Work out the finished part from the listing and answer in its coordinate system (mm). A direction names the side the tool comes from. Coordinates: 2 decimals unless noted, no trailing zeros. Order: outer loops, then holes, each group sorted by start corner. A loop starts at its lowest first (then second) coordinate and runs counter-clockwise, first axis right, second up. Notation, with made-up numbers: M 66,-19.5 L 98,-19.5 A17 cw 98,-0.5 Z; hole C 28,43 d7. An arc over 180 degrees is marked long. Use a Markdown table: item, result.
from build123d import *

# Parameters (mm, degrees)
SKETCH1_R           = 9.2
BOSS_EXTRUDE1_DEPTH = 65
CUT_EXTRUDE2_START  = -3
SKETCH2_R           = 9.2
SKETCH2_R_2         = 7.5
CUT_EXTRUDE2_DEPTH  = 3
CUT_EXTRUDE3_START  = -1.5
SKETCH3_R           = 9.2
SKETCH3_R_2         = 8.419577465
CUT_EXTRUDE3_DEPTH  = 1.5


with BuildPart() as part:
    # Sketch1 → Boss-Extrude1 (new body)
    with BuildSketch(Plane.XY):
        Circle(SKETCH1_R)
    extrude(amount=BOSS_EXTRUDE1_DEPTH)

    # Sketch2 → Cut-Extrude2 (cut)
    with BuildSketch(Plane.XY.offset(65).offset(CUT_EXTRUDE2_START)):
        Circle(SKETCH2_R)
        Circle(SKETCH2_R_2, mode=Mode.SUBTRACT)
    extrude(amount=CUT_EXTRUDE2_DEPTH, mode=Mode.SUBTRACT)

    # Sketch3 → Cut-Extrude3 (cut)
    with BuildSketch(Plane.XY.offset(58).offset(CUT_EXTRUDE3_START)):
        Circle(SKETCH3_R)
        Circle(SKETCH3_R_2, mode=Mode.SUBTRACT)
    extrude(amount=CUT_EXTRUDE3_DEPTH, mode=Mode.SUBTRACT)


solid = part.part
1. Flat-ended cylindrical pins translate along their axes: P1, Ø10, axis at x = -6, z = 54, coming from the -Y side; P2, Ø5, axis at y = -6.5, z = 45.5, coming from the +X side; P3, Ø8, axis at y = -6, z = 35.5, coming from the +X side. Find the tip coordinate at first contact, or state that the pin passes through.
Answers below:
| item | result |
|---|---|
| P1 | y = -9.15 |
| P2 | x = 8.28 |
| P3 | x = 8.98 |
2. For a pull along Z with two mould halves and no side action, classify faces 3 (the face through (0, 0, 0)), 4 (the face through (-7.3, -5.6, 60)), 5 (the face through (8.03, 2.53, 57.24)) as +Z half, -Z half, draft (parallel to the pull), parting line (faces both ways), or undercut.
Answers below:
| item | result |
|---|---|
| face 3 | -Z half |
| face 4 | draft |
| face 5 | undercut |
3. Find the intervals of material crossed by probe 1 along Z at (x, y) = (-7.5, -5); probe 2 along X at (y, z) = (-0.5, 9.5); probe 3 along X at (y, z) = (-7.5, 3.5), in increasing order.
Answers below:
| item | result |
|---|---|
| probe 1 | 0 to 56.5, 58 to 62 |
| probe 2 | -9.19 to 9.19 |
| probe 3 | -5.33 to 5.33 |
4. Section B-B on x = -1.5 is taken. Determine the outline of the cut face in (y, z), then the cut area to 3 significant figures.
Answers below:
| item | result |
|---|---|
| outline | M -9.08,0 L 9.08,0 L 9.08,56.5 L 8.28,56.5 L 8.28,58 L 9.08,58 L 9.08,62 L 7.35,62 L 7.35,65 L -7.35,65 L -7.35,62 L -9.08,62 L -9.08,58 L -8.28,58 L -8.28,56.5 L -9.08,56.5 Z |
| area | 1,170 mm² |
5. Section C-C on z = 53 is taken. Determine the outline of the cut face in (x, y).
Answers below:
| item | result |
|---|---|
| outline | C 0,0 d18.4 |
6. For faces 1 (the face through (0, 0, 65)), 2 (the face through (-7.493, 0.33, 63.479)), determine the directions among +Z, -Z, +X, -X, +Y, -Y from which every point of the face is accessible in a straight line to the end or side of a thin tool.
Answers below:
| item | result |
|---|---|
| face 1 | +Z, +X, -X, +Y, -Y |
| face 2 | +Z |
7. Section A-A on y = 2 is taken. Determine the outline of the cut face in (x, z).
Answers below:
| item | result |
|---|---|
| outline | M -8.98,0 L 8.98,0 L 8.98,56.5 L 8.18,56.5 L 8.18,58 L 8.98,58 L 8.98,62 L 7.23,62 L 7.23,65 L -7.23,65 L -7.23,62 L -8.98,62 L -8.98,58 L -8.18,58 L -8.18,56.5 L -8.98,56.5 Z |
